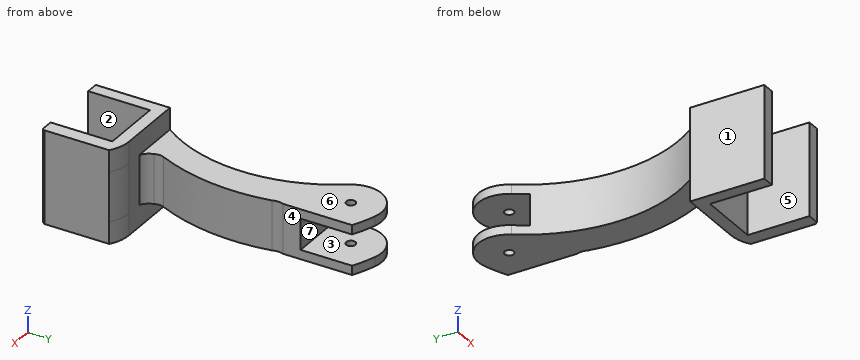
Autodesk Inventor part; units mm, degrees
ref_plane "РабПлоскость1" through (-5.8357, 87.5184, 30) normal (-1, 0, 0) x (0, 0, 1)
ref_plane "РабПлоскость2" through (0, 0, 15) normal (0, 0, -1) x (-1, 0, 0)
ref_plane "YZ Plane" through (0, 0, 0) normal (1, 0, 0) x (0, 1, 0)
sketch "Эскиз1" plane through (0, 0, 0) normal (0, 0, 1) x (1, 0, 0)
  line L0 (0, 0) -> (20, 0) construction
  line L1 (20, 0) -> (20, 20) construction
  line L2 (20, 20) -> (0, 20) construction
  line L3 (0, 20) -> (0, 0) construction
  line L4 (0, 0) -> (0, 20)
  line L5 (0, 0) -> (-4, 0)
  line L6 (-4, 0) -> (-4, 24)
  line L7 (-4, 24) -> (24, 24)
  line L8 (24, 24) -> (24, 0)
  line L9 (24, 0) -> (20, 0)
  line L10 (20, 0) -> (20, 20)
  line L11 (20, 20) -> (0, 20)
  dimension "d0" = 20
  dimension "d1" = 4
  dimension "d2" = 4
extrude "Выдавливание1" add sketch "Эскиз1" along normal blind 30
sketch "Эскиз2" plane through (0, 0, 30) normal (0, 0, 1) x (1, 0, 0)
  line L0 (24, 0) -> (24, 24)
  arc A0 (24, 0) -> (38.6, 61.3222) centre (-41.6488, 48.0293) ccw
  arc A1 (38.6, 61.3222) -> (7.0088, 97.1053) centre (-5.7899, 53.9692) ccw
  line L1 (-4, 24) -> (-4, 0)
  arc A2 (-4, 24) -> (-4, 81.744) centre (-44.8217, 52.872) ccw
  arc A3 (7.0088, 97.1053) -> (-4, 81.744) centre (4.1643, 87.5184) ccw
  circle A4 centre (4.1643, 87.5184) radius 1.5
  line L2 (24, 24) -> (-4, 24)
  point P0 (0, 0)
  dimension "d5" = 10
  dimension "d6" = 3
  dimension "d7" = 50
extrude "Выдавливание2" add sketch "Эскиз2" against normal up to surface (30 mm away)
ref_plane "РабПлоскость1" through (-5.8357, 87.5184, 30) normal (-1, 0, 0) x (0, 0, 1)
sketch "Эскиз4" plane through (-5.8357, 87.5184, 30) normal (-1, 0, 0) x (0, 0, 1)
  line L0 (-20, 10) -> (-10, 10)
  line L1 (-10, 10) -> (-10, -10)
  line L2 (-10, -10) -> (-20, -10)
  line L3 (-20, -10) -> (-20, 10)
  line L4 (0, 10) -> (-30, 10)
  point P0 (-30, -87.5184)
  point P1 (-15, 10)
  dimension "d10" = 10
  dimension "d11" = 20
extrude "Выдавливание3" cut sketch "Эскиз4" against normal through all
sketch "Эскиз5" plane through (-5.8357, 87.5184, 30) normal (-1, 0, 0) x (0, 0, 1)
  line L0 (-30, -26.1962) -> (-30, -87.5184)
  line L1 (-30, -63.5184) -> (-23, -63.5184)
  line L2 (-23, -63.5184) -> (-23, -16.5184)
  line L3 (-23, -16.5184) -> (-30, -16.5184)
  line L4 (-30, -16.5184) -> (-30, -63.5184)
  line L5 (-30, -63.5184) -> (0, -63.5184)
  dimension "d14" = 7
  dimension "d15" = 47
extrude "Выдавливание4" cut sketch "Эскиз5" against normal through all
ref_plane "РабПлоскость2" through (0, 0, 15) normal (0, 0, -1) x (-1, 0, 0)
mirror "Зеркальное отражение1" about plane through (0, 0, 15) normal (0, 0, -1) of "Выдавливание4"
fillet "Сопряжение1" radius 12 2 edges at (36.0633, 24, 3.5) (36.0633, 24, 26.5)
fillet "Сопряжение2" radius 12 2 edges at (35.8572, 71, 3.5) (35.8572, 71, 26.5)
sketch "Эскиз6" plane through (-4, 24, 23) normal (0, 0, 1) x (1, 0, 0)
  arc A0 (17, 4.7391) -> (22, 45) centre (-43.2292, 32.6599) ccw construction
  arc A1 (20.3144, 3.2026) -> (25.5896, 45.6791) centre (-43.2292, 32.6599) ccw
  arc A2 (13.6856, 6.2756) -> (18.4104, 44.3209) centre (-43.2292, 32.6599) ccw
  arc A3 (13.6856, 6.2756) -> (20.3144, 3.2026) centre (17, 4.7391) ccw
  arc A4 (25.5896, 45.6791) -> (18.4104, 44.3209) centre (22, 45) ccw
  line L0 (0, 0) -> (0, -24)
  point P0 (4, -24)
  dimension "d20" = 17
  dimension "d21" = 45
  dimension "d22" = 22
extrude "Выдавливание5" cut sketch "Эскиз6" against normal through all
sketch "Эскиз7" plane through (-4, 24, 23) normal (0, 0, 1) x (1, 0, 0)
  arc A0 (31.8516, -18.235) -> (42.6, 37.3222) centre (-37.6488, 24.0293) ccw
  arc A1 (31.8516, -18.235) -> (21.5986, 0) centre (21.5986, -12) ccw
  arc A2 (42.6, 37.3222) -> (19.593, 69.5583) centre (-1.7899, 29.9692) ccw
  arc A3 (13.8903, 47) -> (19.593, 69.5583) centre (13.8903, 59) ccw
  arc A4 (13.6856, 6.2756) -> (18.4104, 44.3209) centre (-43.2292, 32.6599) ccw
  arc A5 (13.8903, 47) -> (19.593, 69.5583) centre (13.8903, 59) ccw
  arc A6 (18.4174, 47.8867) -> (19.593, 69.5583) centre (13.9238, 58.9982) ccw
  line L0 (0, 0) -> (21.5986, 0)
  arc A7 (13.9667, 6.8907) -> (21.5986, 0) centre (18.8905, 4.6723) ccw
  arc A8 (18.4174, 47.8867) -> (18.4104, 44.3209) centre (22.8221, 46.0952) ccw
  point P0 (4, -24)
  point P1 (19.6658, 69.519)
  point P2 (16.1824, 0)
extrude "Выдавливание6" cut sketch "Эскиз7" against normal blind 36 contours A1 L0 A7 A4 A8 A6 A2 A0
sketch "Эскиз8" plane through (-4, 0, 0) normal (-1, 0, 0) x (0, 0, 1)
  point P0 (0, 0)
sketch "Эскиз9" plane through (-5.8357, 87.5184, 30) normal (-1, 0, 0) x (0, 0, 1)
  line L0 (-23, -16.5184) -> (-23, -63.5184)
  line L1 (-23, -16.5184) -> (-46.8016, -16.5184)
  line L2 (-46.8016, -16.5184) -> (-46.8016, 17.3569)
  line L3 (-46.8016, 17.3569) -> (-23, 17.3569)
  line L4 (-23, 17.3569) -> (-23, -16.5184)
  point P0 (-30, -87.5184)
extrude "Выдавливание7" cut sketch "Эскиз9" against normal blind 36
mirror "Зеркальное отражение2" about plane through (0, 0, 15) normal (0, 0, -1) of "Выдавливание7"
sketch "Эскиз10" plane through (0, 0, 30) normal (0, 0, 1) x (1, 0, 0)
  line L0 (24.5745, 0) -> (35.4567, 0)
  line L1 (35.4567, 0) -> (35.4567, 28.8198)
  line L2 (35.4567, 28.8198) -> (24.5745, 28.8198)
  line L3 (24.5745, 28.8198) -> (24.5745, 0)
  point P0 (0, 0)
extrude "Выдавливание8" cut sketch "Эскиз10" against normal through all
sketch "Эскиз11" plane through (-44.8217, 52.872, 23) normal (0, 0, 1) x (1, 0, 0)
  arc A0 (59.2391, 19.0147) -> (60.4874, 40.647) centre (54.7454, 30.1262) ccw
  line L0 (59.2391, 19.0147) -> (70.8374, 19.0147)
  line L1 (70.8374, 19.0147) -> (70.8374, 43.6051)
  line L2 (70.8374, 43.6051) -> (59.2391, 43.6051)
  line L3 (59.2391, 43.6051) -> (59.2391, 19.0147)
  point P0 (44.8217, -52.872)
extrude "Выдавливание9" cut sketch "Эскиз11" against normal through all
properties part number "shok_absorber_holder"
Work out the finished part from the listing and answer in its coordinate system (mm). Face numbers are marked on the shaded views. A direction names the side the tool comes from. Give positions to 0.01 mm unless a question says otherwise; leave off trailing zeros. Write each loop counter-clockwise with the first axis right and the second up, starting at its lowest first coordinate (ties: lowest second). Pieces come first, ordered by that corner, then holes.
(1) Which of the six approach directions +Z, -Z, +X, -X, +Y, -Y give full straight-line access (tool end or side, diameter ignored) to the marked faces 1, 2, 3 and 4?
Final values:
face 1: +Z, -Z, -X, -Y
face 2: +Z, -Z, -Y
face 3: +X, -X, +Y
face 4: +Z, -Z, +X, +Y
(2) The part is cut by section A-A on y = 15. Write down the section's boundary in (x, z), plus the area to 3 significant figures.
Final values:
outline: (-4, 0) - (0, 0) - (0, 30) - (-4, 30) - close; (20, 0) - (24.57, 0) - (24.57, 30) - (20, 30) - close
area: 257 mm2
(3) The part is cut by section B-B on z = 4. Write down the section's boundary in (x, y).
Final values:
outline: (-4, 0) - (0, 0) - (0, 20) - (20, 20) - (20, 0) - (24, 0) arc R81.34 ccw to (24.57, 0.8) - (24.57, 21.76) arc R12 ccw to (17.6, 24) - (-4, 24) - close
(4) The part is cut by section D-D on z = 22. Write down the section's boundary in (x, y), plus the area to 3 significant figures.
Final values:
outline: (-4, 0) - (0, 0) - (0, 20) - (20, 20) - (20, 0) - (24, 0) arc R81.34 ccw to (24.57, 0.8) - (24.57, 21.76) arc R12 ccw to (17.6, 24) - (12.18, 24) arc R5.4 cw to (9.71, 27.16) arc R3.65 cw to (9.69, 30.28) arc R62.73 ccw to (14.41, 68.32) arc R4.76 cw to (14.42, 71.89) - (14.42, 94.17) arc R44.99 ccw to (7.01, 97.11) arc R10 ccw to (-4, 81.74) arc R50 cw to (-4, 24) - close; hole circle Ø3 at (4.16, 87.52)
area: 1,220 mm2
(5) The part is cut by section C-C on y = 79. Write down the section's boundary in (x, z), plus the area to 3 significant figures.
Final values:
outline: (-2.19, 7) - (14.42, 7) - (14.42, 10) - (-2.19, 10) - close; (-2.19, 20) - (14.42, 20) - (14.42, 23) - (-2.19, 23) - close
area: 99.7 mm2
(6) Flat-ended cylindrical pins translate along their axes: pin 1 Ø12 at (x, y) = (2.5, 35) entering from -Z; pin 2 Ø1 at (x, z) = (20.5, 8.5) entering from +Y; pin 3 Ø6 at (y, z) = (9.5, 11) entering from -X. Find the tip coordinate at first contact, or state that the pin passes through.
Final values:
pin 1: stops at z = 7
pin 2: stops at y = 23.76
pin 3: stops at x = -4
(7) Straight lines are drawn through the part: line 1 (Z direction, x = 10, y = 85); line 2 (X direction, y = 13.5, z = 6); line 3 (Y direction, x = 4, z = 27.5). For each, find the intervals that lie inside material, in ascending order.
Final values:
line 1: z = 7 to 10, 20 to 23
line 2: x = -4 to 0, 20 to 24.57
line 3: y = 20 to 24
(8) The mould has two halves that part along Z. Classify the marked faces 5, 6 and 7: pulls with the +Z half, pulls with the -Z half, needs draft (parallel to the pull), parting line crosses it, or undercut.
Final values:
face 5: needs draft
face 6: pulls with the +Z half
face 7: undercut
